from build123d import *

# Parameters (mm, degrees)
SKETCH1_R           = 1.5875
SKETCH1_R_2         = 1.587499999
BOSS_EXTRUDE1_DEPTH = 3.175


with BuildPart() as part:
    # Sketch1 → Boss-Extrude1 (new body)
    with BuildSketch(Plane(origin=(0, 0, 0), x_dir=(1, 0, 0), z_dir=(0, 1, 0))):
        with BuildLine():
            Line((-19.05, 152.4), (-29.160477546, 70.399620377))
            Line((-29.160477546, 70.399620377), (-24.300397955, 58.666350314))
            ThreePointArc((-24.300397955, 58.666350314), (0, 63.5), (24.300397955, 58.666350314))
            Line((24.300397955, 58.666350314), (29.160477546, 70.399620377))
            Line((29.160477546, 70.399620377), (19.05, 152.4))
            ThreePointArc((19.05, 152.4), (0, 171.45), (-19.05, 152.4))
        make_face()
        with Locations(Location((0, 139.7, 0), (0, 0, 270))):
            Circle(SKETCH1_R, mode=Mode.SUBTRACT)
        with Locations(Location((-12.7, 152.4, 0), (0, 0, 270))):
            Circle(SKETCH1_R, mode=Mode.SUBTRACT)
        with Locations(Location((0, 69.85, 0), (0, 0, 270))):
            Circle(SKETCH1_R, mode=Mode.SUBTRACT)
        with Locations(Location((18.0785103, 67.469918962, 0), (0, 0, 270))):
            Circle(SKETCH1_R, mode=Mode.SUBTRACT)
        with Locations(Location((0, 165.1, 0), (0, 0, 270))):
            Circle(SKETCH1_R, mode=Mode.SUBTRACT)
        with Locations(Location((12.7, 152.4, 0), (0, 0, 270))):
            Circle(SKETCH1_R, mode=Mode.SUBTRACT)
        with Locations(Location((-18.078510302, 67.469918971, 0), (0, 0, 270))):
            Circle(SKETCH1_R_2, mode=Mode.SUBTRACT)
        with BuildLine():
            Line((-15.438109232, 129.802746381), (-4.504911756, 76.066719201))
            ThreePointArc((-4.504911756, 76.066719201), (-13.582616579, 74.97968076), (-22.464793382, 72.813275289))
            Line((-22.464793382, 72.813275289), (-15.438109232, 129.802746381))
        make_face(mode=Mode.SUBTRACT)
        with BuildLine():
            Line((-10.294399454, 136.371031229), (0, 85.774659025))
            Line((0, 85.774659025), (10.294399454, 136.371031229))
            ThreePointArc((10.294399454, 136.371031229), (0, 133.35), (-10.294399454, 136.371031229))
        make_face(mode=Mode.SUBTRACT)
        with BuildLine():
            Line((12.296722124, 155.575), (3.175, 155.575))
            Line((3.175, 155.575), (3.175, 164.696722124))
            ThreePointArc((3.175, 164.696722124), (8.980256121, 161.380256121), (12.296722124, 155.575))
        make_face(mode=Mode.SUBTRACT)
        with BuildLine():
            Line((-3.175, 149.225), (-12.296722124, 149.225))
            ThreePointArc((-12.296722124, 149.225), (-8.980256121, 143.419743879), (-3.175, 140.103277876))
            Line((-3.175, 140.103277876), (-3.175, 149.225))
        make_face(mode=Mode.SUBTRACT)
        with BuildLine():
            Line((12.296722124, 149.225), (3.175, 149.225))
            Line((3.175, 149.225), (3.175, 140.103277876))
            ThreePointArc((3.175, 140.103277876), (8.980256121, 143.419743879), (12.296722124, 149.225))
        make_face(mode=Mode.SUBTRACT)
        with BuildLine():
            Line((4.504911756, 76.066719201), (15.438109232, 129.802746381))
            Line((15.438109232, 129.802746381), (22.464793382, 72.813275289))
            ThreePointArc((22.464793382, 72.813275289), (13.582616579, 74.97968076), (4.504911756, 76.066719201))
        make_face(mode=Mode.SUBTRACT)
        with BuildLine():
            Line((-3.175, 155.575), (-3.175, 164.696722124))
            ThreePointArc((-3.175, 164.696722124), (-8.980256121, 161.380256121), (-12.296722124, 155.575))
            Line((-12.296722124, 155.575), (-3.175, 155.575))
        make_face(mode=Mode.SUBTRACT)
    extrude(amount=BOSS_EXTRUDE1_DEPTH)


solid = part.part
Here's how the part is built. I have some questions about the finished solid (model axes, mm). A direction names the side the tool comes from. Give positions to 0.01 mm unless a question says otherwise; leave off trailing zeros. Loops run counter-clockwise (first coordinate to the right, second up) from the corner with the lowest first, then second, coordinate; pieces in that order, holes last. Notation, with made-up numbers: (78.25, -4) -> (110.25, -4) arc R25 ccw to (110.25, 32) -> close; hole circle Ø5 at (-12.75, 62.5). An arc over 180 degrees is marked (long way). Answer as a JSON object with one key per item and string values. Group by question number.
Item 1: Imagine slicing it at B-B on z = -159. Write out the boundary of the cut face in (x, y) (3 decimals).
Item 2: Imagine slicing it at A-A on z = -126. Write out the boundary of the cut face in (x, y) (3 decimals), then the cut area to 3 significant figures.
Item 3: I need wall thicknesses on L1, parallel to X at y = 1.4, z = -152.4; L2, parallel to X at y = 2.85, z = -87; L3, parallel to X at y = 1.95, z = -115.5. Which ranges of each line are inside material? Lowest first, please.
Item 4: Imagine slicing it at C-C on x = 8. Write out the boundary of the cut face in (y, z) (3 decimals).
Item 5: On a 3-axis mill with a long thin cutter (end or side, diameter ignored), from which of +Z, -Z, +X, -X, +Y, -Y can I reach the whole of each face in a straight line? I mean faces 1 (the flat face through (-8, 2, -149.225)), 2 (the flat face through (26.696, 1.565, -64.451)). Say none if no direction works.
Item 6: Thinking about a two-plate mould opening in X: for faces 3 (the flat face through (-26.764, 1.565, -64.615)), 4 (the flat face through (24.176, 1.565, -110.826)), 5 (the flat face through (18.9, 1.57, -101.71)), 6 (the flat face through (6, 0, -103)), which applies, pulls with the +X half, pulls with the -X half, needs draft (parallel to the pull), parting line crosses it, or undercut?
Item 7: Imagine slicing it at D-D on y = 2. Give the number of separate pieces and of enclosed holes in the cut face, then the cut area to 3 significant figures.
Item 8: Will these pins go through, and if not, where does the flat tip stop? pin 1 (1 mm diameter, centred on y = 2, z = -142.5, fed in from -X); pin 2 (5 mm diameter, centred on x = -14.5, z = -110, fed in from +Y); pin 3 (1 mm diameter, centred on y = 2, z = -146.5, fed in from -X); pin 4 (1.5 mm diameter, centred on y = 0.5, z = -118, fed in from +X).
Answer list:
{
 "1": {"outline": "(-17.87, 0) -> (-10.85, 0) -> (-10.85, 3.175) -> (-17.87, 3.175) -> close; (-3.175, 0) -> (3.175, 0) -> (3.175, 3.175) -> (-3.175, 3.175) -> close; (10.85, 0) -> (17.87, 0) -> (17.87, 3.175) -> (10.85, 3.175) -> close"},
 "2": {"outline": "(-22.305, 0) -> (-15.907, 0) -> (-15.907, 3.175) -> (-22.305, 3.175) -> close; (-14.664, 0) -> (-8.184, 0) -> (-8.184, 3.175) -> (-14.664, 3.175) -> close; (8.184, 0) -> (14.664, 0) -> (14.664, 3.175) -> (8.184, 3.175) -> close; (15.907, 0) -> (22.305, 0) -> (22.305, 3.175) -> (15.907, 3.175) -> close", "area": "81.8 mm2"},
 "3": {"L1": "x = -19.05 to -14.29, -11.11 to 11.11, 14.29 to 19.05", "L2": "x = -27.11 to -20.72, -6.73 to -0.25, 0.25 to 6.73, 20.72 to 27.11", "L3": "x = -23.6 to -17.2, -12.53 to -6.05, 6.05 to 12.53, 17.2 to 23.6"},
 "4": {"outline": "(0, -169.689) -> (3.175, -169.689) -> (3.175, -162.264) -> (0, -162.264) -> close; (0, -155.575) -> (3.175, -155.575) -> (3.175, -149.225) -> (0, -149.225) -> close; (0, -142.536) -> (3.175, -142.536) -> (3.175, -135.111) -> (0, -135.111) -> close; (0, -125.094) -> (3.175, -125.094) -> (3.175, -93.245) -> (0, -93.245) -> close; (0, -75.779) -> (3.175, -75.779) -> (3.175, -62.994) -> (0, -62.994) -> close"},
 "5": {"face 1": "+Y, -Y", "face 2": "+Z, +X, +Y, -Y"},
 "6": {"face 3": "pulls with the -X half", "face 4": "pulls with the +X half", "face 5": "undercut", "face 6": "needs draft"},
 "7": {"separate pieces": "1", "enclosed holes": "14", "area": "3,240 mm2"},
 "8": {"pin 1": "stops at x = -20.33", "pin 2": "passes through", "pin 3": "stops at x = -19.84", "pin 4": "stops at x = 23.38"}
}
